from build123d import *

# Parameters (mm, degrees)
BOSS_EXTRUDE1_DEPTH = 6.35
SKETCH2_R           = 5.08
SKETCH2_R_2         = 3.81
BOSS_EXTRUDE2_DEPTH = 12.7
SKETCH3_R           = 5.715
BOSS_EXTRUDE3_DEPTH = 19.05
SKETCH4_R           = 7.937190451
BOSS_EXTRUDE4_DEPTH = 2.54
SKETCH5_R           = 3.81
CUT_EXTRUDE1_DEPTH  = 26.4
CUT_EXTRUDE2_DEPTH  = 10.16
CIRPATTERN1_COUNT   = 6


with BuildPart() as part:
    # Sketch1 → Boss-Extrude1 (new body)
    with BuildSketch(Plane.XY):
        Polygon((0, 8.248891971), (-7.14375, 4.124445986), (-7.14375, -4.124445986), (0, -8.248891971), (7.14375, -4.124445986), (7.14375, 4.124445986), align=None)
    extrude(amount=BOSS_EXTRUDE1_DEPTH)

    # Sketch2 → Boss-Extrude2 (add)
    with BuildSketch(Plane.XY.offset(6.35)):
        Circle(SKETCH2_R)
        Circle(SKETCH2_R_2, mode=Mode.SUBTRACT)
    extrude(amount=BOSS_EXTRUDE2_DEPTH)

    # Sketch3 → Boss-Extrude3 (add)
    with BuildSketch(Plane(origin=(0, 0, 0), x_dir=(-1, 0, 0), z_dir=(0, 0, -1))):
        Circle(SKETCH3_R)
    extrude(amount=BOSS_EXTRUDE3_DEPTH)

    # Sketch4 → Boss-Extrude4 (add)
    with BuildSketch(Plane(origin=(0, 0, -1.397), x_dir=(-1, 0, 0), z_dir=(0, 0, -1))):
        Circle(SKETCH4_R)
    extrude(amount=BOSS_EXTRUDE4_DEPTH)

    # Sketch5 → Cut-Extrude1 (cut, through all)
    with BuildSketch(Plane.XY.offset(6.35)):
        Circle(SKETCH5_R)
    extrude(amount=-CUT_EXTRUDE1_DEPTH, mode=Mode.SUBTRACT)

    # Sketch6 → Cut-Extrude2 (cut)
    with BuildSketch(Plane.XY.offset(19.05)):
        Polygon((-0.818654099, 4.743933512), (0.818654099, 4.743933512), (1.27, 5.195279413), (-1.27, 5.195279413), align=None)
    cut_extrude2 = extrude(amount=-CUT_EXTRUDE2_DEPTH, mode=Mode.SUBTRACT)

    # CirPattern1: Cut-Extrude2 ×6 about axis
    cirpattern1_axis = Axis((0, 0, 0), (0, 0, 1))
    for i in range(1, CIRPATTERN1_COUNT):
        add(cut_extrude2.rotate(cirpattern1_axis, i * 360 / CIRPATTERN1_COUNT), mode=Mode.SUBTRACT)


solid = part.part
Could you check a few things on this model? Use its own coordinates, in mm. A direction names the side the tool comes from. Give positions to 0.01 mm unless a question says otherwise; leave off trailing zeros. Write each loop counter-clockwise with the first axis right and the second up, starting at its lowest first coordinate (ties: lowest second). Pieces come first, ordered by that corner, then holes. Notation, with made-up numbers: (26.25, 78) -> (30.25, 78) arc R25 cw to (30.25, 105) -> close; hole circle Ø6 at (45, 31.5). An arc over 180 degrees is marked (long way). Answer as a JSON object with one key per item and string values.
Q1. Suppose I cut it at C-C on x = -1.5. Write out the boundary of the cut face in (y, z).
Taken from the geometry:
{"outline": "(-7.79, -3.94) -> (-5.51, -3.94) -> (-5.51, -19.05) -> (-3.5, -19.05) -> (-3.5, 19.05) -> (-4.85, 19.05) -> (-4.85, 6.35) -> (-7.38, 6.35) -> (-7.38, 0) -> (-5.51, 0) -> (-5.51, -1.4) -> (-7.79, -1.4) -> close; (3.5, -19.05) -> (5.51, -19.05) -> (5.51, -3.94) -> (7.79, -3.94) -> (7.79, -1.4) -> (5.51, -1.4) -> (5.51, 0) -> (7.38, 0) -> (7.38, 6.35) -> (4.85, 6.35) -> (4.85, 19.05) -> (3.5, 19.05) -> close"}
Q2. Suppose I cut it at D-D on z = -5. Write out the boundary of the cut face in (x, y) (3 decimals), then the cut area to 3 significant figures.
Taken from the geometry:
{"outline": "circle Ø11.43 at (0, 0); hole circle Ø7.62 at (0, 0)", "area": "57.0 mm²"}
Q3. Suppose I cut it at B-B on y = 0. Write out the boundary of the cut face in (x, z) (3 decimals), then the cut area to 3 significant figures.
Taken from the geometry:
{"outline": "(-7.937, -3.937) -> (-5.715, -3.937) -> (-5.715, -19.05) -> (-3.81, -19.05) -> (-3.81, 19.05) -> (-5.08, 19.05) -> (-5.08, 6.35) -> (-7.144, 6.35) -> (-7.144, 0) -> (-5.715, 0) -> (-5.715, -1.397) -> (-7.937, -1.397) -> close; (3.81, -19.05) -> (5.715, -19.05) -> (5.715, -3.937) -> (7.937, -3.937) -> (7.937, -1.397) -> (5.715, -1.397) -> (5.715, 0) -> (7.144, 0) -> (7.144, 6.35) -> (5.08, 6.35) -> (5.08, 19.05) -> (3.81, 19.05) -> close", "area": "158 mm²"}
Q4. Suppose I cut it at A-A on z = 15. Write out the boundary of the cut face in (x, y).
Taken from the geometry:
{"outline": "(-4.83, -1.58) -> (-4.52, -1.66) -> (-3.7, -3.08) -> (-3.78, -3.39) arc R5.08 ccw to (-1.05, -4.97) -> (-0.82, -4.74) -> (0.82, -4.74) -> (1.05, -4.97) arc R5.08 ccw to (3.78, -3.39) -> (3.7, -3.08) -> (4.52, -1.66) -> (4.83, -1.58) arc R5.08 ccw to (4.83, 1.58) -> (4.52, 1.66) -> (3.7, 3.08) -> (3.78, 3.39) arc R5.08 ccw to (1.05, 4.97) -> (0.82, 4.74) -> (-0.82, 4.74) -> (-1.05, 4.97) arc R5.08 ccw to (-3.78, 3.39) -> (-3.7, 3.08) -> (-4.52, 1.66) -> (-4.83, 1.58) arc R5.08 ccw to start; hole circle Ø7.62 at (0, 0)"}
Q5. Will these pins go through, and if not, where does the flat tip stop? pin 1 Ø5 at (y, z) = (-1, 4.5) entering from +X; pin 2 Ø3 at (x, z) = (-3.5, 8.5) entering from +Y; pin 3 Ø4 at (x, z) = (1.5, 8.5) entering from +Y; pin 4 Ø8 at (x, y) = (0, -2) entering from -Z.
Taken from the geometry:
{"pin 1": "stops at x = 7.14", "pin 2": "stops at y = 4.67", "pin 3": "stops at y = 5.08", "pin 4": "stops at z = -19.05"}
Q6. Which directions (+Z, -Z, +X, -X, +Y, -Y) give clear straight access to the entire face, cutting with the end or side of a thin tool? Please do faces 4 (the flat face through (7.144, 0, 3)), 5 (the flat face through (0, -4.744, 14)), 6 (the flat face through (-5, -2, 6.35)), 7 (the flat face through (3.62, 6.16, 3.13)), 8 (the flat face through (-5.2, -3.4, -1.397)).
Taken from the geometry:
{"face 4": "+Z, +X, +Y, -Y", "face 5": "+Z, -Y", "face 6": "+Z", "face 7": "+Z, +X, +Y", "face 8": "none"}
Q7. Please list where these lines run through material, in increasing order: L1, parallel to Z at x = 0, y = -6; L2, parallel to Y at x = 0, z = -10.75 (3 decimals); L3, parallel to Y at x = 0, z = 14.5.
Taken from the geometry:
{"L1": "z = -3.94 to -1.4, 0 to 6.35", "L2": "y = -5.715 to -3.81, 3.81 to 5.715", "L3": "y = -4.74 to -3.81, 3.81 to 4.74"}
Q8. We'd pull the mould along Z, two halves only. Please class faces 1 (the flat face through (4.3, -2.4, 8.89)), 2 (the flat face through (4.103, 2.382, 14.041)), 3 (the cylindrical face through (-5.45, 1.72, -0.69)): released by +Z, released by -Z, zero draft, split by the parting line, or undercut.
Taken from the geometry:
{"face 1": "released by +Z", "face 2": "zero draft", "face 3": "undercut"}
